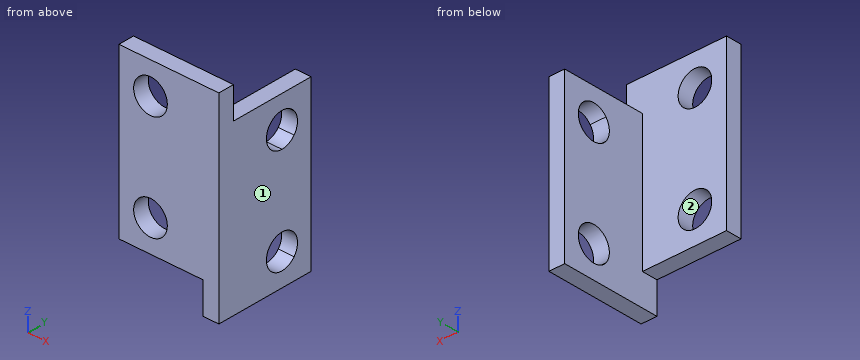
```python
from build123d import *

# Parameters (mm, degrees)
SKETCH1_R           = 1.6
BOSS_EXTRUDE2_DEPTH = 1.5
SKETCH3_W           = 1.5
SKETCH3_H           = 21
BOSS_EXTRUDE3_DEPTH = 8
SKETCH4_R           = 1.6
CUT_EXTRUDE2_DEPTH  = 8
SKETCH6_W           = 5
SKETCH6_H           = 8
CUT_EXTRUDE3_DEPTH  = 8
SKETCH7_W           = 8
SKETCH7_H           = 5
CUT_EXTRUDE4_DEPTH  = 8
SKETCH8_R           = 1.6
SKETCH8_W           = 2
SKETCH8_H           = 9.5
CUT_EXTRUDE5_DEPTH  = 1.5
BOSS_EXTRUDE4_DEPTH = 1.5


with BuildPart() as part:
    # Sketch1 → Boss-Extrude2 (new body)
    with BuildSketch(Plane(origin=(0, 0, 0), x_dir=(1, 0, 0), z_dir=(0, 1, 0))):
        Polygon((-3, 8), (-3, -13), (0, -13), (6.5, -13), (6.5, 0), (6.5, 8), (0, 8), align=None)
        Circle(SKETCH1_R, mode=Mode.SUBTRACT)
        with Locations((0, -10)):
            Circle(SKETCH1_R, mode=Mode.SUBTRACT)
    extrude(amount=BOSS_EXTRUDE2_DEPTH)

    # Sketch3 → Boss-Extrude3 (add)
    with BuildSketch(Plane(origin=(0, 1.5, 0), x_dir=(1, 0, 0), z_dir=(0, 1, 0))):
        with Locations((5.75, -2.5)):
            Rectangle(SKETCH3_W, SKETCH3_H)
    extrude(amount=BOSS_EXTRUDE3_DEPTH)

    # Sketch4 → Cut-Extrude2 (cut)
    with BuildSketch(Plane.ZY.offset(-5)):
        with Locations((-5, 6.5)):
            Circle(SKETCH4_R)
        with Locations((5, 6.5)):
            Circle(SKETCH4_R)
    extrude(amount=-CUT_EXTRUDE2_DEPTH, mode=Mode.SUBTRACT)

    # Sketch6 → Cut-Extrude3 (cut)
    with BuildSketch(Plane.ZY.offset(-5)):
        with Locations((10.5, 5.5)):
            Rectangle(SKETCH6_W, SKETCH6_H)
    extrude(amount=-CUT_EXTRUDE3_DEPTH, mode=Mode.SUBTRACT)

    # Sketch7 → Cut-Extrude4 (cut)
    with BuildSketch(Plane(origin=(0, 1.5, 0), x_dir=(1, 0, 0), z_dir=(0, 1, 0))):
        with Locations((1, 5.5)):
            Rectangle(SKETCH7_W, SKETCH7_H)
    extrude(amount=-CUT_EXTRUDE4_DEPTH, mode=Mode.SUBTRACT)

    # Sketch8 → Cut-Extrude5 (cut)
    with BuildSketch(Plane(origin=(6.5, 0, 0), x_dir=(0, 0, -1), z_dir=(1, 0, 0))):
        with Locations((-7, 6.5)):
            Circle(SKETCH8_R)
        with Locations((3, 6.5)):
            Circle(SKETCH8_R)
        with Locations((7, 4.75)):
            Rectangle(SKETCH8_W, SKETCH8_H)
    extrude(amount=-CUT_EXTRUDE5_DEPTH, mode=Mode.SUBTRACT)

    # Sketch9 → Boss-Extrude4 (add)
    with BuildSketch(Plane(origin=(6.5, 0, 0), x_dir=(0, 0, -1), z_dir=(1, 0, 0))):
        with BuildLine():
            Line((-8, 7.7489996), (-8, 9.5))
            Line((-8, 9.5), (-10, 9.5))
            Line((-10, 9.5), (-10, 1.5))
            Line((-10, 1.5), (-8, 1.5))
            Line((-8, 1.5), (-8, 5.2510004))
            ThreePointArc((-8, 5.2510004), (-8.6, 6.5), (-8, 7.7489996))
        make_face()
        with BuildLine():
            ThreePointArc((-6, 5.2510004), (-3.4, 6.5), (-6, 7.7489996))
            ThreePointArc((-6, 7.7489996), (-5.55777949, 7.192820323), (-5.4, 6.5))
            ThreePointArc((-5.4, 6.5), (-5.55777949, 5.807179677), (-6, 5.2510004))
        make_face()
        with BuildLine():
            ThreePointArc((4, 5.2510004), (4.6, 6.5), (4, 7.7489996))
            ThreePointArc((4, 7.7489996), (5, 8.1), (6, 7.7489996))
            Line((6, 7.7489996), (6, 5.2510004))
            ThreePointArc((6, 5.2510004), (5, 4.9), (4, 5.2510004))
        make_face()
        with BuildLine():
            Line((6, 0), (6, 5.2510004))
            ThreePointArc((6, 5.2510004), (5, 4.9), (4, 5.2510004))
            ThreePointArc((4, 5.2510004), (1.4, 6.5), (4, 7.7489996))
            ThreePointArc((4, 7.7489996), (5, 8.1), (6, 7.7489996))
            Line((6, 7.7489996), (6, 9.5))
            Line((6, 9.5), (-8, 9.5))
            Line((-8, 9.5), (-8, 7.7489996))
            ThreePointArc((-8, 7.7489996), (-7, 8.1), (-6, 7.7489996))
            ThreePointArc((-6, 7.7489996), (-3.4, 6.5), (-6, 5.2510004))
            ThreePointArc((-6, 5.2510004), (-7, 4.9), (-8, 5.2510004))
            Line((-8, 5.2510004), (-8, 1.5))
            Line((-8, 1.5), (-13, 1.5))
            Line((-13, 1.5), (-13, 0))
            Line((-13, 0), (6, 0))
        make_face()
    extrude(amount=-BOSS_EXTRUDE4_DEPTH)


solid = part.part
```
Here's how the part is built. I have some questions about the finished solid (model axes, mm). Face numbers are marked on the shaded views. Coordinates: 2 decimals unless noted, no trailing zeros. Order: outer loops, then holes, each group sorted by start corner. A loop starts at its lowest first (then second) coordinate and runs counter-clockwise, first axis right, second up. Notation, with made-up numbers: M 78,21 L 91,21 A15 cw 91,33 Z; hole C -28.5,38 d8. An arc over 180 degrees is marked long. Answer as a JSON object with one key per item and string values. Group by question number.
(1) For pin 1 (1.9 mm diameter, centred on y = 6.5, z = -3, fed in from +X); pin 2 (1.6 mm diameter, centred on x = 0.5, y = 1, fed in from -Z); pin 3 (5 mm diameter, centred on x = 0, z = 10, fed in from +Y); pin 4 (1.5 mm diameter, centred on y = 3, z = -2.5, fed in from -X), each with a flat end and sliding along its axis, tell me the tip position at first contact or that it passes through.
(2) Suppose I cut it at B-B, the plane y = 1.25. Please give me the cut outline in (x, z).
(3) Suppose I cut it at D-D, the plane y = 5.5. Please give me the cut outline in (x, z).
(4) I need wall thicknesses on probe 1 along Z at (x, y) = (0, 0.3); probe 2 along X at (y, z) = (1.05, 10); probe 3 along Y at (x, z) = (0.5, 2). Which ranges of each line are inside material? Lowest first, please.
(5) If we mould it in two halves opening along Z, with no side actions, what happens to the marked faces 1 and 2? For each: released by +Z, released by -Z, zero draft, split by the parting line, or undercut.
(6) Suppose I cut it at C-C, the plane z = 11. Please give me the cut outline in (x, y), then the cut area to 3 significant figures.
(7) Suppose I cut it at A-A, the plane x = 0. Please give me the cut outline in (y, z), then the cut area to 3 significant figures.
Values found:
{
 "1": {"pin 1": "passes through", "pin 2": "stops at z = -3", "pin 3": "stops at y = 1.5", "pin 4": "stops at x = 5"},
 "2": {"outline": "M -3,-3 L 5,-3 L 5,-6 L 6.5,-6 L 6.5,13 L -3,13 Z; hole C 0,0 d3.2; hole C 0,10 d3.2"},
 "3": {"outline": "M 5,-6 L 6.5,-6 L 6.5,-4.25 L 5,-4.25 Z; M 5,-1.75 L 6.5,-1.75 L 6.5,5.75 L 5,5.75 Z; M 5,8.25 L 6.5,8.25 L 6.5,10 L 5,10 Z"},
 "4": {"probe 1": "z = -3 to -1.6, 1.6 to 8.4, 11.6 to 13", "probe 2": "x = -3 to -1.6, 1.6 to 6.5", "probe 3": "y = 0 to 1.5"},
 "5": {"face 1": "zero draft", "face 2": "undercut"},
 "6": {"outline": "M -3,0 L -1.25,0 L -1.25,1.5 L -3,1.5 Z; M 1.25,0 L 6.5,0 L 6.5,1.5 L 1.25,1.5 Z", "area": "10.5 mm^2"},
 "7": {"outline": "M 0,-3 L 1.5,-3 L 1.5,-1.6 L 0,-1.6 Z; M 0,1.6 L 1.5,1.6 L 1.5,8.4 L 0,8.4 Z; M 0,11.6 L 1.5,11.6 L 1.5,13 L 0,13 Z", "area": "14.4 mm^2"}
}
